Build history of the part. All positions in model axes, mm. A direction names the side the tool comes from. Round coordinates to 2 decimals unless told otherwise and drop trailing zeros. Write each loop counter-clockwise with the first axis right and the second up, starting at its lowest first coordinate (ties: lowest second). Pieces come first, ordered by that corner, then holes. Notation, with made-up numbers: (44.25, 77) -> (92.25, 77) arc R20 ccw to (92.25, 90) -> close; hole circle Ø4 at (75, 5.5). An arc over 180 degrees is marked (long way). Answer in a Markdown table with one row per item. Add a question column.
from build123d import *

# Parameters (mm, degrees)
SKETCH_219_W        = 62.5
SKETCH_219_H        = 20.18
EXTRUDE_1_DEPTH     = 40.57
SKETCH_6_W          = 15.25
SKETCH_6_H          = 20.18
CUT_EXTRUDE_1_DEPTH = 2.55
SKETCH_7_R          = 1.5
CUT_EXTRUDE_2_DEPTH = 15
SKETCH_8_R          = 1.5
EXTRUDE_2_DEPTH     = 4
CHAMFER_1_SIZE      = 5
CHAMFER_2_SIZE      = 5


with BuildPart() as part:
    # Sketch 219 → Бобышка-Вытянуть1 (new body)
    with BuildSketch(Plane(origin=(0, 0, 0), x_dir=(1, 0, 0), z_dir=(0, 1, 0))):
        Rectangle(SKETCH_219_W, SKETCH_219_H)
    extrude(amount=EXTRUDE_1_DEPTH)

    # Эскиз6 → Вырез-Вытянуть1 (cut)
    with BuildSketch(Plane(origin=(0, 40.57, 0), x_dir=(1, 0, 0), z_dir=(0, 1, 0))):
        with Locations((-19.375, 0)):
            Rectangle(SKETCH_6_W, SKETCH_6_H)
    extrude(amount=-CUT_EXTRUDE_1_DEPTH, mode=Mode.SUBTRACT)

    # Эскиз7 → Вырез-Вытянуть2 (cut)
    with BuildSketch(Plane(origin=(0, 40.57, 0), x_dir=(1, 0, 0), z_dir=(0, 1, 0))):
        with BuildLine():
            ThreePointArc((27.3, 0), (25.8, 1.5), (24.3, 0))
            Line((24.3, 0), (27.3, 0))
        make_face()
        with BuildLine():
            Line((27.3, 0), (24.3, 0))
            ThreePointArc((24.3, 0), (25.8, -1.5), (27.3, 0))
        make_face()
        with Locations(Location((11.87, 0, 0), (0, 0, 270))):
            Circle(SKETCH_7_R)
    extrude(amount=-CUT_EXTRUDE_2_DEPTH, mode=Mode.SUBTRACT)

    # Эскиз8 → Бобышка-Вытянуть2 (add)
    # profile 1 of 2: a face of its own
    with BuildSketch(Plane.XZ):
        with BuildLine():
            Line((-31.25, 5.59), (-42.25, 5.59))
            ThreePointArc((-42.25, 5.59), (-45.078427125, 4.418427125), (-46.25, 1.59))
            Line((-46.25, 1.59), (-46.25, -2.41))
            ThreePointArc((-46.25, -2.41), (-45.078427125, -5.238427125), (-42.25, -6.41))
            Line((-42.25, -6.41), (-31.25, -6.41))
            Line((-31.25, -6.41), (-31.25, 5.59))
        make_face()
        with Locations(Location((-40.25, -0.41, 0), (0, 0, 270))):
            Circle(SKETCH_8_R, mode=Mode.SUBTRACT)
    # profile 2 of 2: a face of its own
    with BuildSketch(Plane.XZ):
        with BuildLine():
            Line((31.25, -6.41), (42.25, -6.41))
            ThreePointArc((42.25, -6.41), (45.078427125, -5.238427125), (46.25, -2.41))
            Line((46.25, -2.41), (46.25, 1.59))
            ThreePointArc((46.25, 1.59), (45.078427125, 4.418427125), (42.25, 5.59))
            Line((42.25, 5.59), (31.25, 5.59))
            Line((31.25, 5.59), (31.25, -6.41))
        make_face()
        with Locations(Location((40.25, -0.41, 0), (0, 0, 90))):
            Circle(SKETCH_8_R, mode=Mode.SUBTRACT)
    extrude(amount=-EXTRUDE_2_DEPTH)

    # Фаска1
    chamfer_1_edges = [part.edges().sort_by_distance(p)[0] for p in [
        (-31.25, 4, -0.41),
    ]]
    chamfer(chamfer_1_edges, length=CHAMFER_1_SIZE)

    # Фаска2
    chamfer_2_edges = [part.edges().sort_by_distance(p)[0] for p in [
        (31.25, 4, -0.41),
    ]]
    chamfer(chamfer_2_edges, length=CHAMFER_2_SIZE)


solid = part.part
(1) Saw through at A-A (x = 40.25). List the corners of the cut face in (y, z), plus the area to 3 significant figures.
(2) Saw through at D-D (x = 11.87). List the corners of the cut face in (y, z), plus the area to 3 significant figures.
(3) Saw through at B-B (z = 0). Count the separate pieces of the cut face and the enclosed holes in it, plus the area to 3 significant figures.
(4) Drop flat-ended pins along their axis: P1, Ø1, axis at y = 7, z = -1, coming from the +X side; P2, Ø12, axis at x = -9, z = 8, coming from the -Y side; P3, Ø6, axis at y = 30.5, z = -6.5, coming from the -X side; P4, Ø5, axis at x = 40.5, z = 2, coming from the +Y side. Give the stop position or say it passes through.
(5) Saw through at C-C (y = 31.5). List the corners of the cut face in (x, z), plus the area to 3 significant figures.
(6) Probe line 1 along X through (y, z) = (2.85, -0.41); line 2 along X through (y, z) = (38.5, 3.5); line 3 along Z through (x, y) = (-40, 1). List the from-to ranges inside material, lowest first.
(7) Which spindle directions (+Z, -Z, +X, -X, +Y, -Y) get a long thin tool onto all of the face, cutting with end or side? Do faces 1 (the face through (13.357, 33.175, -0.195)), 2 (the face through (36, 2, 5.59)), 3 (the face through (-19, 38.02, 0)), 4 (the face through (-35, 2, 5.59)). Say none if no direction does.
(8) Mould opens along Z. For faces 5 (the face through (-41.3, 4, 1)), 6 (the face through (26, 25.57, 0)), 7 (the face through (45.047, 1.972, -5.269)) say: pulls with the +Z half, pulls with the -Z half, needs draft (parallel to the pull), parting line crosses it, or undercut.
Answer sheet:
| question | item | result |
|---|---|---|
| 1 | outline | (0, -6.41) -> (4, -6.41) -> (4, -1.91) -> (0, -1.91) -> close; (0, 1.09) -> (4, 1.09) -> (4, 5.59) -> (0, 5.59) -> close |
| 1 | area | 36.0 mm² |
| 2 | outline | (0, -10.09) -> (40.57, -10.09) -> (40.57, -1.5) -> (25.57, -1.5) -> (25.57, 1.5) -> (40.57, 1.5) -> (40.57, 10.09) -> (0, 10.09) -> close |
| 2 | area | 774 mm² |
| 3 | separate pieces | 3 |
| 3 | enclosed holes | 0 |
| 3 | area | 2,530 mm² |
| 4 | P1 | stops at x = 33.75 |
| 4 | P2 | stops at y = 0 |
| 4 | P3 | stops at x = -31.25 |
| 4 | P4 | stops at y = 4 |
| 5 | outline | (-31.25, -10.09) -> (31.25, -10.09) -> (31.25, 10.09) -> (-31.25, 10.09) -> close; hole circle Ø3 at (11.87, 0); hole circle Ø3 at (25.8, 0) |
| 5 | area | 1,250 mm² |
| 6 | line 1 | x = -46.25 to -41.75, -38.75 to 38.75, 41.75 to 46.25 |
| 6 | line 2 | x = -31.25 to -27, -11.75 to 31.25 |
| 6 | line 3 | z = -6.41 to -1.89, 1.07 to 5.59 |
| 7 | face 1 | +Y |
| 7 | face 2 | +Z, +X, +Y, -Y |
| 7 | face 3 | +Z, -Z, +Y |
| 7 | face 4 | +Z, -X, +Y, -Y |
| 8 | face 5 | needs draft |
| 8 | face 6 | undercut |
| 8 | face 7 | pulls with the -Z half |
